The figure shows three views and two pictorial views of one solid part (mm, origin at its lowest corner). Answer the questions. Coordinates: 2 decimals unless noted, no trailing zeros. Order: outer loops, then holes, each group sorted by start corner. A loop starts at its lowest first (then second) coordinate and runs counter-clockwise, first axis right, second up. Notation, with made-up numbers: (84, 50.5) -> (136, 50.5) arc R14 ccw to (136, 60.5) -> close; hole circle Ø3 at (20, 25.25). An arc over 180 degrees is marked (long way). Return JSON: item names as keys, results as strings.
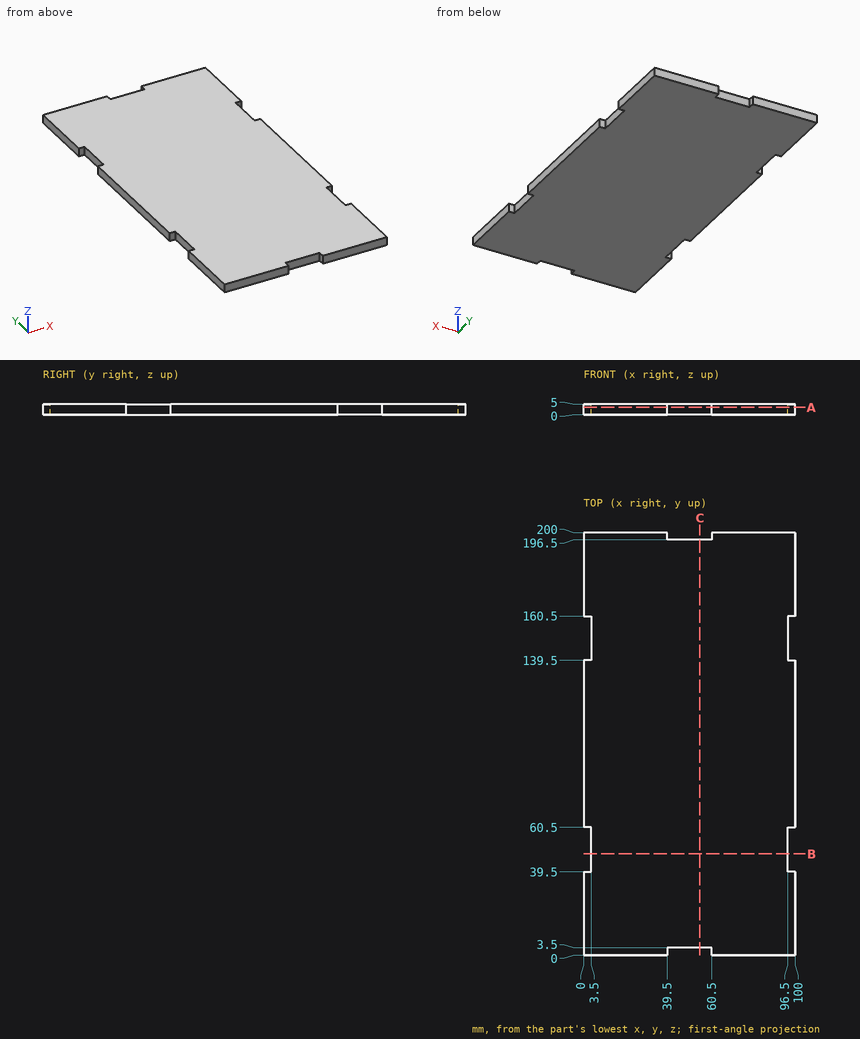
Item 1: The part is cut by section A-A on z = 3.35. Determine the outline of the cut face in (x, y), plus the area to 3 significant figures.
Answer list:
{"outline": "(0, 0) -> (39.5, 0) -> (39.5, 3.5) -> (60.5, 3.5) -> (60.5, 0) -> (100, 0) -> (100, 39.5) -> (96.5, 39.5) -> (96.5, 60.5) -> (100, 60.5) -> (100, 139.5) -> (96.5, 139.5) -> (96.5, 160.5) -> (100, 160.5) -> (100, 200) -> (60.5, 200) -> (60.5, 196.5) -> (39.5, 196.5) -> (39.5, 200) -> (0, 200) -> (0, 160.5) -> (3.5, 160.5) -> (3.5, 139.5) -> (0, 139.5) -> (0, 60.5) -> (3.5, 60.5) -> (3.5, 39.5) -> (0, 39.5) -> close", "area": "19,600 mm2"}
Item 2: Flat-ended cylindrical pins translate along their axes: pin 1 (1.8 mm diameter, centred on y = 2, z = 2, fed in from -X); pin 2 (2.5 mm diameter, centred on x = 51, z = 2.5, fed in from -Y). Find the tip coordinate at first contact, or state that the pin passes through.
Answer list:
{"pin 1": "x = 0", "pin 2": "y = 3.5"}
Item 3: Find the intervals of material crossed by probe 1 along Y at (x, z) = (51.5, 0.55); probe 2 along X at (y, z) = (57.5, 4.55), in increasing order.
Answer list:
{"probe 1": "3.5 to 196.5", "probe 2": "3.5 to 96.5"}
Item 4: The part is cut by section C-C on x = 55. Determine the outline of the cut face in (y, z), plus the area to 3 significant figures.
Answer list:
{"outline": "(3.5, 0) -> (196.5, 0) -> (196.5, 5) -> (3.5, 5) -> close", "area": "965 mm2"}
Item 5: The part is cut by section B-B on y = 48. Determine the outline of the cut face in (x, z), plus the area to 3 significant figures.
Answer list:
{"outline": "(3.5, 0) -> (96.5, 0) -> (96.5, 5) -> (3.5, 5) -> close", "area": "465 mm2"}
